Here's the drawing with two shaded views (mm, measured from the low corner). I have some questions. A direction names the side the tool comes from. Give positions to 0.01 mm unless a question says otherwise; leave off trailing zeros. Write each loop counter-clockwise with the first axis right and the second up, starting at its lowest first coordinate (ties: lowest second). Pieces come first, ordered by that corner, then holes. Notation, with made-up numbers: (-6.5, -27) - (28.5, -27) arc R35 cw to (28.5, 9) - close; hole circle Ø7 at (-21.5, 24). An arc over 180 degrees is marked (long way). Answer as CSV lines item,"result". Start each with the question number.
Q1. We'd pull the mould along Z, two halves only. Please class the marked faces 1, 2 and 3: pulls with the +Z half, pulls with the -Z half, needs draft (parallel to the pull), parting line crosses it, or undercut.
Q2. If I drill on line 1 along X through (y, z) = (5, 7); line 2 along X through (y, z) = (0.5, 12); line 3 along Z through (x, y) = (8.75, 2.5), over which ranges is the centre line in solid material (lowest first)?
Q3. Imagine slicing it at A-A on y = 1. List the corners of the cut face in (x, z) for me (1 decimal).
Q4. On a 3-axis mill with a long thin cutter (end or side, diameter ignored), from which of +Z, -Z, +X, -X, +Y, -Y can I reach the whole of each face in a straight line? I mean the marked faces 4 and 5. Say none if no direction works.
Q5. Will this pin go through, and if not, where does the flat tip stop? pin 1 Ø3 at (y, z) = (1, 4.5) entering from +X.
Q6. Imagine slicing it at B-B on y = 2.5. List the corners of the cut face in (x, z) for me (1 decimal).
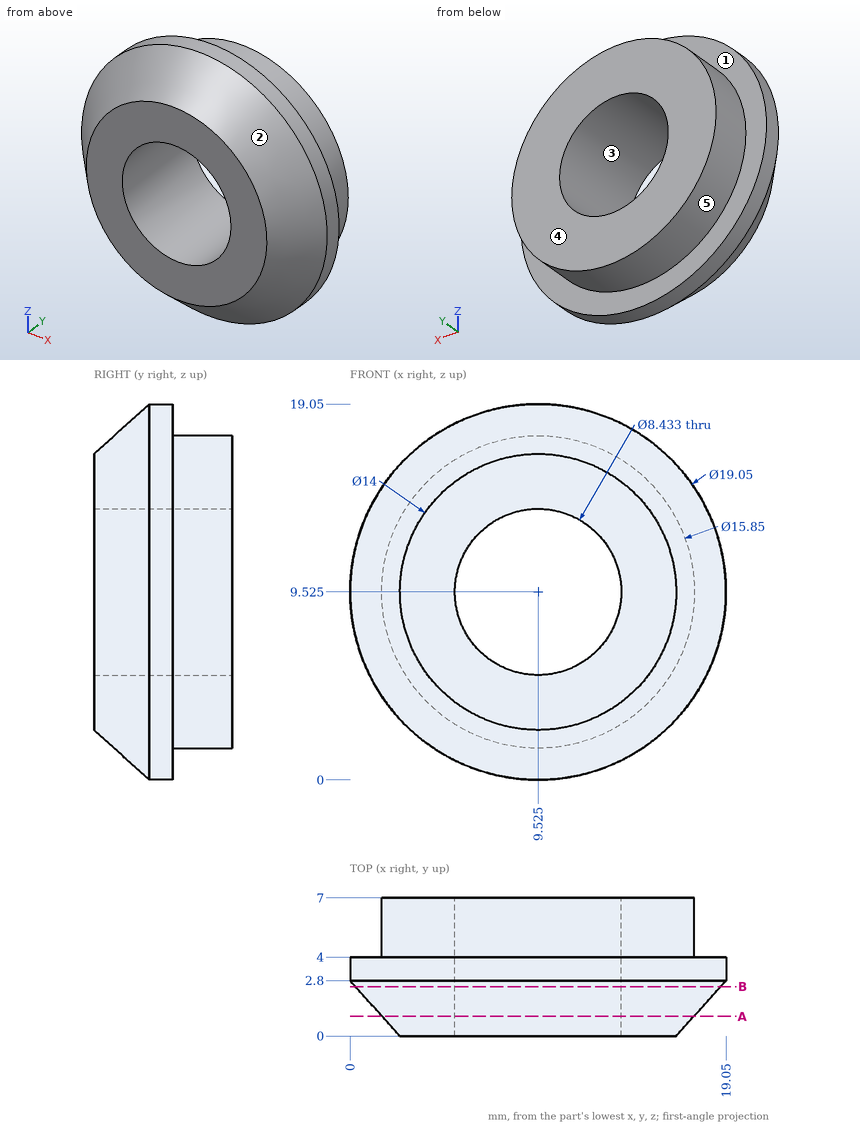
Conclusion:
1,face 1,"needs draft"
1,face 2,"parting line crosses it"
1,face 3,"undercut"
2,line 1,"2.01 to 6.15, 12.9 to 17.04"
2,line 2,"2.5 to 6.11, 12.94 to 16.55"
2,line 3,"0.3 to 5.38, 13.67 to 18.75"
3,outline,"circle Ø15.8 at (9.5, 9.5); hole circle Ø8.4 at (9.5, 9.5)"
4,face 4,"+Z, -Z, +X, -X, +Y"
4,face 5,"+Y"
5,pin 1,"x = 17.53"
6,outline,"circle Ø18.5 at (9.5, 9.5); hole circle Ø8.4 at (9.5, 9.5)"
